```python
from build123d import *

# Parameters (mm, degrees)
SKETCH1_R           = 3.175
BOSS_EXTRUDE1_DEPTH = 6.35


with BuildPart() as part:
    # Sketch1 → Boss-Extrude1 (new body)
    with BuildSketch(Plane.XY):
        with BuildLine():
            Line((6.35, 6.35), (21.59, 19.05))
            ThreePointArc((21.59, 19.05), (44.100663682, 1.273044039), (72.075222755, -5.065267043))
            Line((72.075222755, -5.065267043), (69.85, -6.35))
            Line((69.85, -6.35), (6.35, -6.35))
            Line((6.35, -6.35), (-6.35, -6.35))
            Line((-6.35, -6.35), (-6.35, 6.35))
            Line((-6.35, 6.35), (6.35, 6.35))
        make_face()
        Circle(SKETCH1_R, mode=Mode.SUBTRACT)
        with BuildLine():
            Line((6.35, -3.175), (46.306849943, -3.175))
            ThreePointArc((46.306849943, -3.175), (32.739109843, 4.274408806), (21.204775898, 14.596056128))
            Line((21.204775898, 14.596056128), (6.35, 2.217076213))
            Line((6.35, 2.217076213), (6.35, -3.175))
        make_face(mode=Mode.SUBTRACT)
    extrude(amount=BOSS_EXTRUDE1_DEPTH)


solid = part.part
```
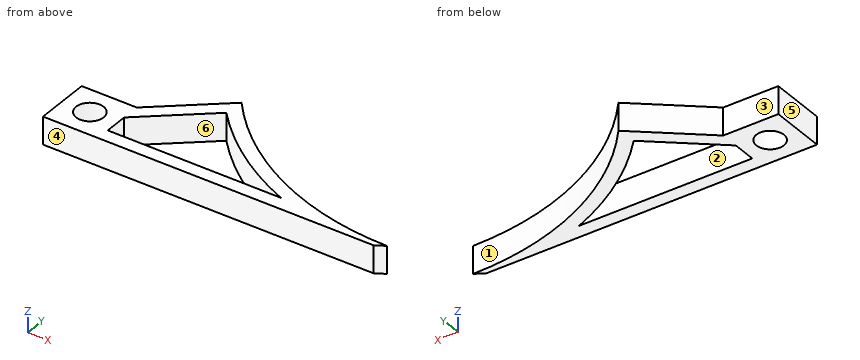
CAD build for the part. Positions are in the model's coordinates, mm. Face numbers are marked on the shaded views. A direction names the side the tool comes from. Round coordinates to 2 decimals unless told otherwise and drop trailing zeros. Loops run counter-clockwise (first coordinate to the right, second up) from the corner with the lowest first, then second, coordinate; pieces in that order, holes last. Notation, with made-up numbers: M 41.25,-31.5 L 85.25,-31.5 A24 ccw 85.25,-2.5 Z; hole C 16,84 d7. An arc over 180 degrees is marked long. Use a Markdown table: item, result. Add a question column.
(1) Flat gauge pins, fed straight in: pin 1 (3 mm diameter, centred on y = 14.5, z = 2, fed in from +X); pin 2 (1 mm diameter, centred on x = 55, z = 5.5, fed in from +Y); pin 3 (1.9 mm diameter, centred on x = 0.5, z = 2.5, fed in from +Y). Where does each tip first touch, or does it go through?
(2) Pull direction Y, two halves, no side cores. Call the marked faces 3, 4, 5 and 6: +Y half, -Y half, draft (parallel to the pull), parting line (faces both ways), or undercut.
(3) Which spindle directions (+Z, -Z, +X, -X, +Y, -Y) get a long thin tool onto all of the face, cutting with end or side? Do the marked faces 1 and 2. Say none if no direction does.
(4) Cut at A-A (z = 4.75). Give the cut face in (x, y) (3 decimals), and give its area (3 significant figures).
(5) Drill centre lines: line 1 (Y direction, x = 0, z = 2) (3 decimals); line 2 (X direction, y = 1.5, z = 3); line 3 (X direction, y = 8.25, z = 3). Where is each one in solid material? Low to high.
(6) Cut at B-B (x = 0). Give the cut face in (y, z) (3 decimals), and give its area (3 significant figures).
(7) Cut at C-C (y = 0). Give the cut face in (x, z) (3 decimals), and give its area (3 significant figures).
(8) Cut at D-D (y = 10.75). Give the cut face in (x, z).
Geometry says:
| question | item | result |
|---|---|---|
| 1 | pin 1 | stops at x = 27.15 |
| 1 | pin 2 | stops at y = -2.64 |
| 1 | pin 3 | stops at y = 6.35 |
| 2 | face 3 | +Y half |
| 2 | face 4 | -Y half |
| 2 | face 5 | draft |
| 2 | face 6 | undercut |
| 3 | face 1 | +Z, -Z, +X, +Y |
| 3 | face 2 | +Z, -Z |
| 4 | outline | M -6.35,-6.35 L 69.85,-6.35 L 72.075,-5.065 A64.903 cw 21.59,19.05 L 6.35,6.35 L -6.35,6.35 Z; hole C 0,0 d6.35; hole M 6.35,-3.175 L 46.307,-3.175 A68.078 cw 21.205,14.596 L 6.35,2.217 Z |
| 4 | area | 494 mm² |
| 5 | line 1 | y = -6.35 to -3.175, 3.175 to 6.35 |
| 5 | line 2 | x = -6.35 to -2.8, 2.8 to 6.35, 36.99 to 43.63 |
| 5 | line 3 | x = 8.63 to 13.59, 27.65 to 32.69 |
| 6 | outline | M -6.35,0 L -3.175,0 L -3.175,6.35 L -6.35,6.35 Z; M 3.175,0 L 6.35,0 L 6.35,6.35 L 3.175,6.35 Z |
| 6 | area | 40.3 mm² |
| 7 | outline | M -6.35,0 L -3.175,0 L -3.175,6.35 L -6.35,6.35 Z; M 3.175,0 L 6.35,0 L 6.35,6.35 L 3.175,6.35 Z; M 39.609,0 L 46.939,0 L 46.939,6.35 L 39.609,6.35 Z |
| 7 | area | 86.9 mm² |
| 8 | outline | M 11.63,0 L 16.59,0 L 16.59,6.35 L 11.63,6.35 Z; M 24.91,0 L 29.62,0 L 29.62,6.35 L 24.91,6.35 Z |
